Could you check a few things on this model? Use its own coordinates, in mm. A direction names the side the tool comes from. Coordinates: 2 decimals unless noted, no trailing zeros. Write each loop counter-clockwise with the first axis right and the second up, starting at its lowest first coordinate (ties: lowest second). Pieces come first, ordered by that corner, then holes.
```python
from build123d import *

# Parameters (mm, degrees)
CROQUIS2_R              = 7.5
SALIENTE_EXTRUIR1_DEPTH = 200
CROQUIS3_W              = 20
CROQUIS3_H              = 15
CORTAR_EXTRUIR1_START   = -100
CROQUIS5_R              = 42.5
CORTAR_EXTRUIR1_DEPTH   = 100
CROQUIS6_W              = 20
CROQUIS6_H              = 15
SALIENTE_EXTRUIR2_DEPTH = 10
CROQUIS8_R              = 5
CORTAR_EXTRUIR2_DEPTH   = 231.922064916


with BuildPart() as part:
    # Croquis2 → Saliente-Extruir1 (new body)
    with BuildSketch(Plane(origin=(0, 0, 0), x_dir=(0, 0, -1), z_dir=(1, 0, 0))):
        Circle(CROQUIS2_R)
    extrude(amount=-SALIENTE_EXTRUIR1_DEPTH)

    # Barrer1: sweep along a path in Croquis4
    with BuildLine(Plane.XY) as barrer1_path:
        ThreePointArc((0, 50), (-50, 0), (0, -50))
    # Croquis3 → Barrer1 (sweep)
    with BuildSketch(Plane(origin=(0, 0, 0), x_dir=(0, 0, -1), z_dir=(1, 0, 0))):
        with Locations((0, 50)):
            Rectangle(CROQUIS3_W, CROQUIS3_H)
    sweep(path=barrer1_path.line)

    # Croquis5 → Cortar-Extruir1 (cut)
    with BuildSketch(Plane.XY.offset(10).offset(CORTAR_EXTRUIR1_START)):
        Circle(CROQUIS5_R)
    extrude(amount=CORTAR_EXTRUIR1_DEPTH, mode=Mode.SUBTRACT)

    # Croquis6 → Saliente-Extruir2 (add)
    with BuildSketch(Plane(origin=(0, 0, 0), x_dir=(0, 0, -1), z_dir=(1, 0, 0))):
        with Locations((0, 50)):
            Rectangle(CROQUIS6_W, CROQUIS6_H)
    saliente_extruir2 = extrude(amount=SALIENTE_EXTRUIR2_DEPTH)

    # Simetría1: Saliente-Extruir2 across plane
    add(saliente_extruir2.mirror(Plane.ZX))

    # Croquis8 → Cortar-Extruir2 (cut, through all)
    with BuildSketch(Plane(origin=(0, 57.5, 0), x_dir=(1, 0, 0), z_dir=(0, 1, 0))):
        with Locations(Location((0, 0, 0), (0, 0, 270))):
            Circle(CROQUIS8_R)
    extrude(amount=-CORTAR_EXTRUIR2_DEPTH, mode=Mode.SUBTRACT)


solid = part.part
```
Item 1: I want a section at A-A, the plane z = -1. List the corners of the cut face in (x, y) for me.
Item 2: Which directions (+Z, -Z, +X, -X, +Y, -Y) give clear straight access to the entire face, cutting with the end or side of a thin tool? Please do faces 4 (the flat face through (6, -42.5, 0)), 5 (the flat face through (6, 57.5, 0)).
Item 3: I want a section at B-B, the plane x = -34. List the corners of the cut face in (y, z) for me, then the cut area to 3 significant figures.
Item 4: I want a section at D-D, the plane x = -185.5. List the corners of the cut face in (y, z) for me.
Item 5: If I drill on line 1 along Z through (x, y) = (0, 46); line 2 along X through (y, z) = (49, 0); line 3 along X through (y, z) = (-44, -4), over which ranges is the centre line in solid material (lowest first)?
Item 6: If we mould it in two halves opening along Z, with no side actions, what happens to faces 1 (the cylindrical face through (-127.503, 0.33, 7.493)), 2 (the cylindrical face through (-4.88, 49.96, -1.08)), 3 (the flat face through (6, 42.5, 0))? For each: released by +Z, released by -Z, zero draft, split by the parting line, or undercut.
Item 7: Will these pins go through, and if not, where does the flat tip stop? pin 1 Ø10 at (y, z) = (7.5, 0) entering from +X; pin 2 Ø3 at (x, z) = (-122, 0.5) entering from -Y; pin 3 Ø10 at (x, z) = (-23, -7.5) entering from +Y.
Item 8: I want a section at C-C, the plane y = 0. List the corners of the cut face in (x, z) for me.
Taken from the geometry:
1. outline: (-200, -7.43) - (-57.02, -7.43) arc R57.5 ccw to (-4.9, -57.29) - (-4.9, -42.22) arc R42.5 cw to (-4.9, 42.22) - (-4.9, 57.29) arc R57.5 ccw to (-57.02, 7.43) - (-200, 7.43) - close; (4.9, -57.5) - (10, -57.5) - (10, -42.5) - (4.9, -42.5) - close; (4.9, 42.5) - (10, 42.5) - (10, 57.5) - (4.9, 57.5) - close
2. face 4: +Z, -Z, +X
2. face 5: +Z, -Z, +X, -X, +Y
3. outline: (-46.37, -10) - (-25.5, -10) - (-25.5, 10) - (-46.37, 10) - close; (25.5, -10) - (46.37, -10) - (46.37, 10) - (25.5, 10) - close
3. area: 835 mm2
4. outline: circle Ø15 at (0, 0)
5. line 1: z = -10 to -5, 5 to 10
5. line 2: x = -30.09 to -5, 5 to 10
5. line 3: x = -37.02 to -3, 3 to 10
6. face 1: split by the parting line
6. face 2: undercut
6. face 3: zero draft
7. pin 1: stops at x = -40.62
7. pin 2: stops at y = -7.5
7. pin 3: stops at y = 54.61
8. outline: (-200, -7.5) - (-57.5, -7.5) - (-57.5, -10) - (-42.5, -10) - (-42.5, 10) - (-57.5, 10) - (-57.5, 7.5) - (-200, 7.5) - close
